from build123d import *

# Parameters (mm, degrees)
F1_DEPTH = 30.4
F2_DEPTH = 2
F3_W     = 6.8
F3_H     = 6.8
F4_DEPTH = 50
F5_R     = 1


with BuildPart() as f1:
    # F0 (on Top) → F1 (new body)
    with BuildSketch(Plane.XY):
        with BuildLine():
            ThreePointArc((0, -17), (-17, 0), (0, 17))
            Line((0, 17), (-27.8, 17))
            Line((-27.8, 17), (-27.8, -17))
            Line((-27.8, -17), (0, -17))
        make_face()
        with BuildLine():
            ThreePointArc((0, -16.25), (-16.25, 0), (0, 16.25))
            Line((0, 16.25), (0, 17))
            ThreePointArc((0, 17), (-17, 0), (0, -17))
            Line((0, -17), (0, -16.25))
        make_face()
        with BuildLine():
            ThreePointArc((0, 16.25), (11.4904851943, 11.4904851943), (16.25, 0))
            ThreePointArc((16.25, 0), (11.4904851943, -11.4904851943), (0, -16.25))
            Line((0, -16.25), (0, -17))
            ThreePointArc((0, -17), (12.0208152802, -12.0208152802), (17, 0))
            ThreePointArc((17, 0), (12.0208152802, 12.0208152802), (0, 17))
            Line((0, 17), (0, 16.25))
        make_face()
    extrude(amount=F1_DEPTH)

    # F0 (on Top) → F2 (join)
    with BuildSketch(Plane.XY):
        with BuildLine():
            ThreePointArc((0, -16.25), (11.4904851943, -11.4904851943), (16.25, 0))
            ThreePointArc((16.25, 0), (11.4904851943, 11.4904851943), (0, 16.25))
            Line((0, 16.25), (0, 14.75))
            ThreePointArc((0, 14.75), (1.2374368671, 14.2374368671), (1.75, 13))
            ThreePointArc((1.75, 13), (1.6167891819, 12.3303039934), (1.2374368671, 11.7625631329))
            Line((1.2374368671, 11.7625631329), (4.2019029611, 8.7980970389))
            ThreePointArc((4.2019029611, 8.7980970389), (6.8942911166, 6.8942911166), (8.7980970389, 4.2019029611))
            Line((8.7980970389, 4.2019029611), (11.7625631329, 1.2374368671))
            ThreePointArc((11.7625631329, 1.2374368671), (13.6696960066, 1.6167891819), (14.75, 0))
            ThreePointArc((14.75, 0), (13.6696960066, -1.6167891819), (11.7625631329, -1.2374368671))
            Line((11.7625631329, -1.2374368671), (8.7980970389, -4.2019029611))
            ThreePointArc((8.7980970389, -4.2019029611), (6.8942911166, -6.8942911166), (4.2019029611, -8.7980970389))
            Line((4.2019029611, -8.7980970389), (1.2374368671, -11.7625631329))
            ThreePointArc((1.2374368671, -11.7625631329), (1.6167891819, -12.3303039934), (1.75, -13))
            ThreePointArc((1.75, -13), (1.2374368671, -14.2374368671), (0, -14.75))
            Line((0, -14.75), (0, -16.25))
        make_face()
        with BuildLine():
            Line((0, 14.75), (0, 16.25))
            ThreePointArc((0, 16.25), (-16.25, 0), (0, -16.25))
            Line((0, -16.25), (0, -14.75))
            ThreePointArc((0, -14.75), (-1.6167891819, -13.6696960066), (-1.2374368671, -11.7625631329))
            Line((-1.2374368671, -11.7625631329), (-4.2019029611, -8.7980970389))
            ThreePointArc((-4.2019029611, -8.7980970389), (-6.8942911166, -6.8942911166), (-8.7980970389, -4.2019029611))
            Line((-8.7980970389, -4.2019029611), (-11.7625631329, -1.2374368671))
            ThreePointArc((-11.7625631329, -1.2374368671), (-14.75, 0), (-11.7625631329, 1.2374368671))
            Line((-11.7625631329, 1.2374368671), (-8.7980970389, 4.2019029611))
            ThreePointArc((-8.7980970389, 4.2019029611), (-6.8942911166, 6.8942911166), (-4.2019029611, 8.7980970389))
            Line((-4.2019029611, 8.7980970389), (-1.2374368671, 11.7625631329))
            ThreePointArc((-1.2374368671, 11.7625631329), (-1.6167891819, 13.6696960066), (0, 14.75))
        make_face()
        with BuildLine():
            ThreePointArc((1.2374368671, 11.7625631329), (0.6696960066, 11.3832108181), (0, 11.25))
            Line((0, 11.25), (0, 9.75))
            ThreePointArc((0, 9.75), (2.1541882312, 9.5090469062), (4.2019029611, 8.7980970389))
            Line((4.2019029611, 8.7980970389), (1.2374368671, 11.7625631329))
        make_face()
        with BuildLine():
            ThreePointArc((0, 11.25), (-0.6696960066, 11.3832108181), (-1.2374368671, 11.7625631329))
            Line((-1.2374368671, 11.7625631329), (-4.2019029611, 8.7980970389))
            ThreePointArc((-4.2019029611, 8.7980970389), (-2.1541882312, 9.5090469062), (0, 9.75))
            Line((0, 9.75), (0, 11.25))
        make_face()
        with BuildLine():
            ThreePointArc((-8.7980970389, -4.2019029611), (-9.75, 0), (-8.7980970389, 4.2019029611))
            Line((-8.7980970389, 4.2019029611), (-11.7625631329, 1.2374368671))
            ThreePointArc((-11.7625631329, 1.2374368671), (-11.3832108181, 0.6696960066), (-11.25, 0))
            ThreePointArc((-11.25, 0), (-11.3832108181, -0.6696960066), (-11.7625631329, -1.2374368671))
            Line((-11.7625631329, -1.2374368671), (-8.7980970389, -4.2019029611))
        make_face()
        with BuildLine():
            Line((11.7625631329, 1.2374368671), (8.7980970389, 4.2019029611))
            ThreePointArc((8.7980970389, 4.2019029611), (9.5090469062, 2.1541882312), (9.75, 0))
            ThreePointArc((9.75, 0), (9.5090469062, -2.1541882312), (8.7980970389, -4.2019029611))
            Line((8.7980970389, -4.2019029611), (11.7625631329, -1.2374368671))
            ThreePointArc((11.7625631329, -1.2374368671), (11.25, 0), (11.7625631329, 1.2374368671))
        make_face()
        with BuildLine():
            Line((0, -9.75), (0, -11.25))
            ThreePointArc((0, -11.25), (0.6696960066, -11.3832108181), (1.2374368671, -11.7625631329))
            Line((1.2374368671, -11.7625631329), (4.2019029611, -8.7980970389))
            ThreePointArc((4.2019029611, -8.7980970389), (2.1541882312, -9.5090469062), (0, -9.75))
        make_face()
        with BuildLine():
            Line((-4.2019029611, -8.7980970389), (-1.2374368671, -11.7625631329))
            ThreePointArc((-1.2374368671, -11.7625631329), (-0.6696960066, -11.3832108181), (0, -11.25))
            Line((0, -11.25), (0, -9.75))
            ThreePointArc((0, -9.75), (-2.1541882312, -9.5090469062), (-4.2019029611, -8.7980970389))
        make_face()
    extrude(amount=F2_DEPTH)

    # F3 (on face) → F4 (cut)
    with BuildSketch(Plane.XZ.offset(17)):
        with Locations((-22.4, 25)):
            Rectangle(F3_W, F3_H)
        with Locations((-22.4, 5.4)):
            Rectangle(F3_W, F3_H)
    extrude(amount=-F4_DEPTH, mode=Mode.SUBTRACT)

    # F5
    f5_edges = [f1.edges().sort_by_distance(p)[0] for p in [
        (-27.8, 17, 15.2),
        (-27.8, -17, 15.2),
    ]]
    fillet(f5_edges, radius=F5_R)


solid = f1.part
Verification items for the finished model (mm, model axes). A direction names the side the tool comes from. Coordinates: 2 decimals unless noted, no trailing zeros. Order: outer loops, then holes, each group sorted by start corner. A loop starts at its lowest first (then second) coordinate and runs counter-clockwise, first axis right, second up. Notation, with made-up numbers: (-23, 45) -> (-3, 45) arc R38 cw to (-3, 83) -> close; hole circle Ø2 at (-33, -28). An arc over 180 degrees is marked (long way). Use CSV: the item, a comma, the result in double quotes. Start each with the question number.
Q1. Section check A-A, the plane z = 5. Record the cut outline in (x, y), and give its area (3 significant figures).
Q2. Section check C-C, the plane x = -13. Record the cut outline in (y, z), and give its area (3 significant figures).
Q3. Thickness scan on line 1 along Z through (x, y) = (-23, 10.5); line 2 along X through (y, z) = (2.5, 7); line 3 along Y through (x, z) = (-13, 1). Record the ranges inside material, lowest first.
Q4. Tool access check on faces 4 (the flat face through (-19, 0, 5)), 5 (the flat face through (-27.8, 0, 15)). Record the directions out of +Z, -Z, +X, -X, +Y, -Y that give a thin tool (end or side, any length) a straight path to the whole face; none if there is none.
Q5. Section check B-B, the plane y = -6. Record the cut outline in (x, z).
Q6. Depth check by flat-ended pin: P1, Ø3, axis at x = -13, y = 0, coming from the -Z side; P2, Ø2, axis at y = 2.5, z = 25, coming from the +X side; P3, Ø16, axis at x = -5.5, y = 5.5, coming from the +Z side; P4, Ø1.5, axis at x = 8.5, z = 27, coming from the +Y side. Enter the tip coordinate at first touch or a pass-through.
Q7. Section check D-D, the plane z = 19.5. Record the cut outline in (x, y).
Q8. Draft check along Y on faces 1 (the flat face through (0, -11, 2)), 2 (the flat face through (-22, 0, 28.4)), 3 (the cylindrical face through (-27.515, -16.699, 15.413)). Enter one of: +Y half, -Y half, draft (parallel to the pull), parting line (faces both ways), or undercut.
Returned:
1,outline,"(-27.8, -16) arc R1 ccw to (-26.8, -17) -> (-25.8, -17) -> (-25.8, 17) -> (-26.8, 17) arc R1 ccw to (-27.8, 16) -> close; (-19, -17) -> (0, -17) arc R17 ccw to (0, 17) -> (-19, 17) -> close; hole circle Ø32.5 at (0, 0)"
1,area,"338 mm^2"
2,outline,"(-17, 0) -> (-1.75, 0) -> (-1.75, 2) -> (-9.75, 2) -> (-9.75, 30.4) -> (-17, 30.4) -> close; (1.75, 0) -> (17, 0) -> (17, 30.4) -> (9.75, 30.4) -> (9.75, 2) -> (1.75, 2) -> close"
2,area,"473 mm^2"
3,line 1,"z = 0 to 2, 8.8 to 21.6, 28.4 to 30.4"
3,line 2,"x = -27.8 to -25.8, -19 to -16.06, 16.06 to 16.82"
3,line 3,"y = -17 to -1.75, 1.75 to 17"
4,face 4,"+Y, -Y"
4,face 5,"+Z, -Z, -X, +Y, -Y"
5,outline,"(-27.8, 0) -> (-7.69, 0) -> (-7.69, 2) -> (-15.1, 2) -> (-15.1, 30.4) -> (-27.8, 30.4) -> close; (7.69, 0) -> (15.91, 0) -> (15.91, 30.4) -> (15.1, 30.4) -> (15.1, 2) -> (7.69, 2) -> close; hole (-25.8, 2) -> (-19, 2) -> (-19, 8.8) -> (-25.8, 8.8) -> close; hole (-25.8, 21.6) -> (-19, 21.6) -> (-19, 28.4) -> (-25.8, 28.4) -> close"
6,P1,"passes through"
6,P2,"stops at x = 16.93"
6,P3,"stops at z = 2"
6,P4,"stops at y = 15.13"
7,outline,"(-27.8, -16) arc R1 ccw to (-26.8, -17) -> (0, -17) arc R17 ccw to (0, 17) -> (-26.8, 17) arc R1 ccw to (-27.8, 16) -> close; hole circle Ø32.5 at (0, 0)"
8,face 1,"undercut"
8,face 2,"draft"
8,face 3,"-Y half"
